The model under review builds one solid part; all positions refer to its coordinate system, in mm. Face numbers are marked on the shaded views. Round coordinates to 2 decimals unless told otherwise and drop trailing zeros. Order: outer loops, then holes, each group sorted by start corner. A loop starts at its lowest first (then second) coordinate and runs counter-clockwise, first axis right, second up. Notation, with made-up numbers: (1, 76.5) -> (56, 76.5) arc R8 ccw to (56, 85.5) -> close; hole circle Ø11 at (-29, 57.5). An arc over 180 degrees is marked (long way). Use a Markdown table: item, result. Add a question column.
```python
from build123d import *

# Parameters (mm, degrees)
F0_R           = 19.05
F1_DEPTH       = 69.85
F2_R           = 14
F3_DEPTH       = 30.48
F4_R           = 12.5
F5_DEPTH       = 1
F7_D           = 9.525
F7_CBORE_D     = 12.7
F7_CBORE_DEPTH = 6.35
F8_R           = 9
F9_DEPTH       = 6.35
F11_R          = 14.8971
F11_R_2        = 14
F12_DEPTH      = 2.54
F13_SIZE       = 1.27


with BuildPart() as f1:
    # F0 (on Top) → F1 (new body)
    with BuildSketch(Plane.XY):
        with Locations((-34.2093408108, -25.4185739905)):
            Circle(F0_R)
    extrude(amount=F1_DEPTH)

    # F2 (on face) → F3 (cut)
    with BuildSketch(Plane(origin=(0, 0, 0), x_dir=(1, 0, 0), z_dir=(0, 0, -1))):
        with Locations((-34.2093408108, 25.4185739905)):
            Circle(F2_R)
    extrude(amount=-F3_DEPTH, mode=Mode.SUBTRACT)

    # F4 (on face) → F5 (cut)
    with BuildSketch(Plane(origin=(0, 0, 30.48), x_dir=(1, 0, 0), z_dir=(0, 0, -1))):
        with Locations((-34.2093408108, 25.4185739905)):
            Circle(F4_R)
    extrude(amount=-F5_DEPTH, mode=Mode.SUBTRACT)

    # F7 (through all)
    with Locations(Plane.XY.offset(69.85)):
        with Locations((-34.2093408108, -25.4185739905)):
            CounterBoreHole(F7_D / 2, F7_CBORE_D / 2, F7_CBORE_DEPTH)

    # F8 (on face) → F9 (cut)
    with BuildSketch(Plane(origin=(0, 0, 31.48), x_dir=(1, 0, 0), z_dir=(0, 0, -1))):
        with Locations((-34.2093408108, 25.4185739905)):
            Circle(F8_R)
    extrude(amount=-F9_DEPTH, mode=Mode.SUBTRACT)

    # F11 (on offset) → F12 (cut)
    with BuildSketch(Plane(origin=(0, 0, 2.032), x_dir=(1, 0, 0), z_dir=(0, 0, -1))):
        with Locations((-34.2093408108, 25.4185739905)):
            Circle(F11_R)
        with Locations((-34.2093408108, 25.4185739905)):
            Circle(F11_R_2, mode=Mode.SUBTRACT)
    extrude(amount=-F12_DEPTH, mode=Mode.SUBTRACT)

    # F13
    f13_edges = [f1.edges().sort_by_distance(p)[0] for p in [
        (-53.259341, -25.418574, 69.85),
        (-53.259341, -25.418574, 0),
    ]]
    chamfer(f13_edges, length=F13_SIZE)


solid = f1.part
```
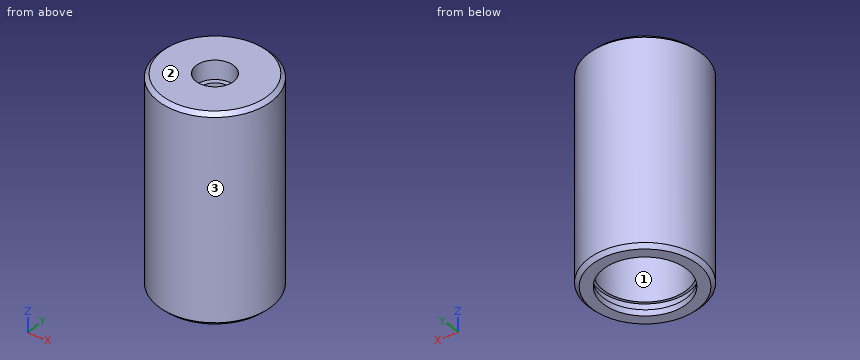
Q1. For pin 1 (12 mm diameter, centred on y = -13, z = 24.5, fed in from +X); pin 2 (10 mm diameter, centred on x = -34.5, z = 42.5, fed in from -Y); pin 3 (3 mm diameter, centred on y = -26.5, z = 7.5, fed in from -X); pin 4 (9 mm diameter, centred on x = -30, y = -26.5, fed in from -Z), all flat-tipped, find the tip position at first contact; note any pin that passes through.
Q2. Add section B-B, the plane z = 6.5. Give the boundary of the cut face in (x, y).
Q3. To check wall thickness, follow line 1 along Z through (x, y) = (-20, -27); line 2 along Z through (x, y) = (-45, -25.5); line 3 along Z through (x, y) = (-28.5, -26). State the ranges of each line that lie inside material, in increasing order.
Q4. Draft analysis for pull direction Y (two halves, no side actions). For the marked faces 1, 2 and 3, state which applies: released by +Y, released by -Y, zero draft, split by the parting line, or undercut.
Return value:
| question | item | result |
|---|---|---|
| 1 | pin 1 | x = -16.27 |
| 1 | pin 2 | y = -44.47 |
| 1 | pin 3 | x = -53.26 |
| 1 | pin 4 | z = 37.83 |
| 2 | outline | circle Ø38.1 at (-34.21, -25.42); hole circle Ø28 at (-34.21, -25.42) |
| 3 | line 1 | 0 to 2.03, 4.57 to 69.85 |
| 3 | line 2 | 31.48 to 69.85 |
| 3 | line 3 | 37.83 to 63.5 |
| 4 | face 1 | undercut |
| 4 | face 2 | zero draft |
| 4 | face 3 | split by the parting line |
